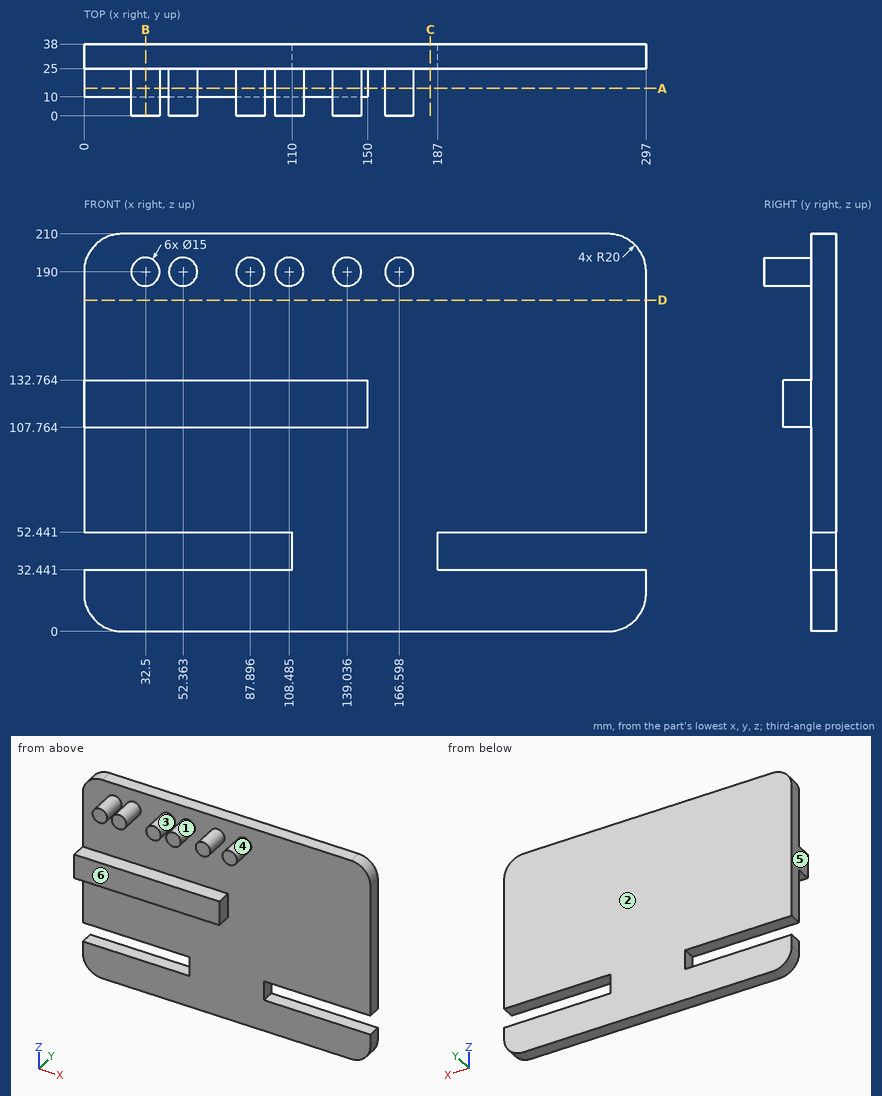
Answer from the drawing. Dimensions are ordinates in mm from the lowest x, y and z of the part. A direction names the side the tool comes from. Round coordinates to 2 decimals unless told otherwise and drop trailing zeros. Write each loop counter-clockwise with the first axis right and the second up, starting at its lowest first coordinate (ties: lowest second). Pieces come first, ordered by that corner, then holes. Notation, with made-up numbers: M -15,82 L 18,82 A24 ccw 18,112 Z; hole C -26.5,-25.5 d10. An arc over 180 degrees is marked long. One line per item, written item: value.
Q1. Which of the six approach directions +Z, -Z, +X, -X, +Y, -Y give full straight-line access (tool end or side, diameter ignored) to the marked faces 1 and 2?
Data:
face 1: -Y
face 2: +Z, -Z, +X, -X, +Y
Q2. Flat-ended cylindrical pins translate along their axes: pin 1 Ø6 at (y, z) = (21.5, 125) entering from +X; pin 2 Ø4 at (y, z) = (29, 43.5) entering from -X; pin 3 Ø7.5 at (x, z) = (70.5, 125.5) entering from -Y; pin 4 Ø16.5 at (x, y) = (58, 20) entering from +Z. Find the tip coordinate at first contact, or state that the pin passes through.
Data:
pin 1: x = 150
pin 2: x = 110
pin 3: y = 10
pin 4: z = 210
Q3. Find section C-C on x = 183. Write down the section's boundary in (y, z).
Data:
outline: M 25,0 L 38,0 L 38,210 L 25,210 Z
Q4. For a pull along X with two mould halves and no side action, classify the marked faces 3, 4, 5 and 6 as +X half, -X half, draft (parallel to the pull), parting line (faces both ways), or undercut.
Data:
face 3: undercut
face 4: undercut
face 5: -X half
face 6: draft
Q5. Find section B-B on x = 32.5. Write down the section's boundary in (y, z), plus the area to 3 significant figures.
Data:
outline: M 0,182.5 L 25,182.5 L 25,132.76 L 10,132.76 L 10,107.76 L 25,107.76 L 25,52.44 L 38,52.44 L 38,210 L 25,210 L 25,197.5 L 0,197.5 Z; M 25,0 L 38,0 L 38,32.44 L 25,32.44 Z
area: 3,220 mm2
Q6. Straight lines are drawn through the part: line 1 (Z direction, x = 193, y = 33.5); line 2 (Z direction, x = 32.5, y = 5); line 3 (Y direction, x = 236, z = 132.5). For each, find the intervals that lie inside material, in ascending order. Write a range as [from, to].
Data:
line 1: [0, 32.44], [52.44, 210]
line 2: [182.5, 197.5]
line 3: [25, 38]
Q7. Find section D-D on z = 175. Write down the section's boundary in (x, y), plus the area to 3 significant figures.
Data:
outline: M 0,25 L 297,25 L 297,38 L 0,38 Z
area: 3,860 mm2
Q8. Find section A-A on y = 14.5. Write down the section's boundary in (x, z) (1 decimal), plus the area to 3 significant figures.
Data:
outline: M 0,107.8 L 150,107.8 L 150,132.8 L 0,132.8 Z; C 32.5,190 d15; C 52.4,190 d15; C 87.9,190 d15; C 108.5,190 d15; C 139,190 d15; C 166.6,190 d15
area: 4,810 mm2
